```python
from build123d import *


with BuildPart() as part:
    # Sketch1 → Revolve1 (revolve)
    with BuildSketch(Plane.XY):
        with BuildLine():
            Line((12.5, 7), (12.5, 139.066923077))
            ThreePointArc((12.5, 139.066923077), (11.964906619, 140.358752773), (10.673076923, 140.893846154))
            Line((10.673076923, 140.893846154), (10, 141.566923077))
            Line((10, 141.566923077), (10.673076923, 142.24))
            Line((10.673076923, 142.24), (11.673076923, 142.24))
            ThreePointArc((11.673076923, 142.24), (13.355924313, 141.034344496), (14, 139.066923077))
            Line((14, 139.066923077), (14, 0))
            Line((14, 0), (15.5, 0))
            Line((15.5, 0), (15.5, -6))
            Line((15.5, -6), (14.5, -6))
            ThreePointArc((14.5, -6), (13.538055577, -2.948361096), (11, -1))
            Line((11, -1), (11, 2))
            Line((11, 2), (10, 2))
            Line((10, 2), (10, 7))
            Line((10, 7), (12.5, 7))
        make_face()
    revolve(axis=Axis((0, -1085.204253018, 0), (0, 1, 0)))


solid = part.part
```
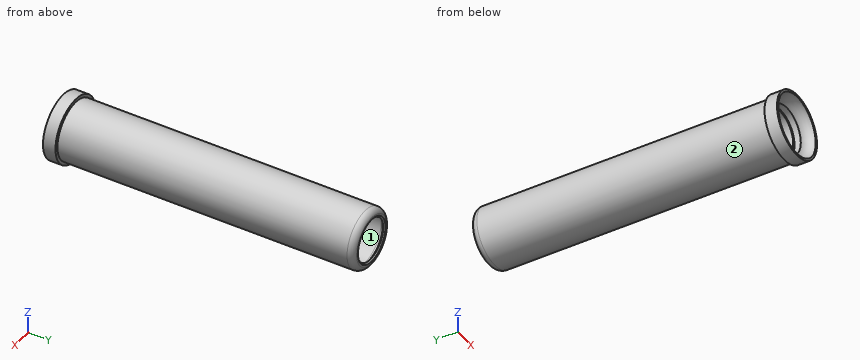
Read the model definition and answer for the solid it produces. Units are mm, in the model's axes. Face numbers are marked on the shaded views. Round coordinates to 2 decimals unless told otherwise and drop trailing zeros. Write each loop counter-clockwise with the first axis right and the second up, starting at its lowest first coordinate (ties: lowest second). Pieces come first, ordered by that corner, then holes. Notation, with made-up numbers: (52.25, 2.25) -> (64.25, 2.25) arc R24 cw to (64.25, 37.25) -> close; hole circle Ø9 at (-39, 73). An arc over 180 degrees is marked (long way). Answer in a Markdown table with one row per item. Add a question column.
1) Find section C-C, the plane y = 61. Determine the outline of the cut face in (x, z).
2) Consider line 1 (Z direction, x = 0, y = 5); line 2 (X direction, y = 102, z = 0); line 3 (Z direction, x = 0, y = -0.2). Determine where each line is inside the solid, lowest interval first.
3) Determine the mould class of the marked faces 1 and 2 for opening direction Z: pulls with the +Z half, pulls with the -Z half, needs draft (parallel to the pull), parting line crosses it, or undercut.
4) Given P1, Ø6.5, axis at x = 3.5, z = 3, coming from the -Y side; P2, Ø5, axis at y = 59.5, z = -2.5, coming from the -X side; P3, Ø5, axis at y = 119, z = -6.5, coming from the +X side; P4, Ø4, axis at x = -3, y = 104, coming from the +Z side, each flat-ended and moving along its own axis, determine where each tip first touches the part or whether it passes through.
Findings below:
| question | item | result |
|---|---|---|
| 1 | outline | circle Ø28 at (0, 0); hole circle Ø25 at (0, 0) |
| 2 | line 1 | -14 to -10, 10 to 14 |
| 2 | line 2 | -14 to -12.5, 12.5 to 14 |
| 2 | line 3 | -15.5 to -11, 11 to 15.5 |
| 3 | face 1 | undercut |
| 3 | face 2 | parting line crosses it |
| 4 | P1 | through |
| 4 | P2 | x = -14 |
| 4 | P3 | x = 13.42 |
| 4 | P4 | z = 13.96 |
